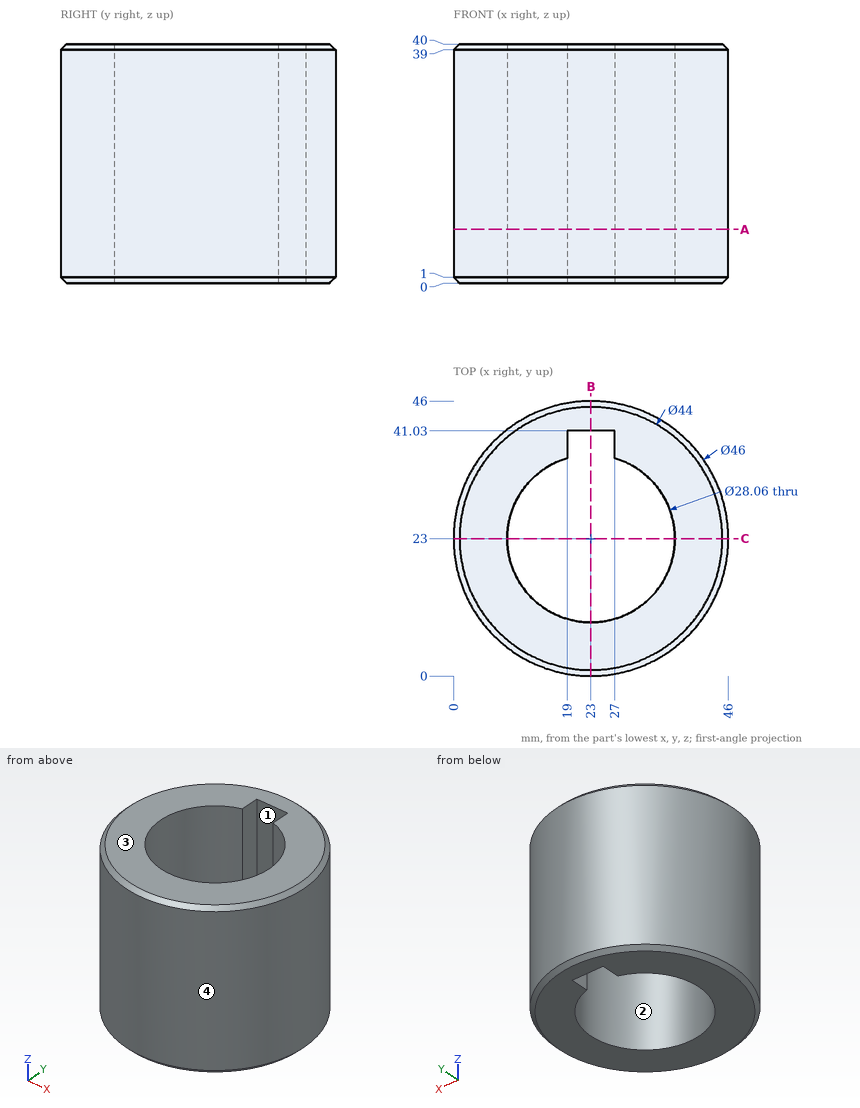
Job drawing, mm, ordinate dimensions from the low corner. One solid piece. Give positions to 0.01 mm unless a question says otherwise; leave off trailing zeros. Loops run counter-clockwise (first coordinate to the right, second up) from the corner with the lowest first, then second, coordinate; pieces in that order, holes last. Notation, with made-up numbers: M 54,64 L 66,64 A12 ccw 66,74 Z; hole C -13.75,24.25 d2. An arc over 180 degrees is marked long. Return JSON: item names as keys, results as strings.
1) Saw through at A-A, the plane z = 9. List the corners of the cut face in (x, y).
Calculated:
{"outline": "C 23,23 d46; hole M 19,36.45 A14.03 ccw long 27,36.45 L 27,41.03 L 19,41.03 Z"}
2) Saw through at C-C, the plane y = 23. List the corners of the cut face in (x, z).
Calculated:
{"outline": "M 0,1 L 1,0 L 8.97,0 L 8.97,40 L 1,40 L 0,39 Z; M 37.03,0 L 45,0 L 46,1 L 46,39 L 45,40 L 37.03,40 Z"}
3) Flat gauge pins, fed straight in: pin 1 Ø2 at (y, z) = (31.5, 12) entering from +X; pin 2 Ø5 at (y, z) = (38, 21.5) entering from +X; pin 3 Ø10 at (y, z) = (16.5, 18.5) entering from -X. Where does each tip first touch, or does it go through?
Calculated:
{"pin 1": "stops at x = 44.74", "pin 2": "stops at x = 42.31", "pin 3": "stops at x = 0.05"}
4) Drill centre lines: line 1 (Y direction, x = 23, z = 31); line 2 (Y direction, x = 29, z = 11.5); line 3 (X direction, y = 22, z = 19.5). Where is each one in solid material? Low to high.
Calculated:
{"line 1": "y = 0 to 8.97, 41.03 to 46", "line 2": "y = 0.8 to 10.32, 35.68 to 45.2", "line 3": "x = 0.02 to 9.01, 36.99 to 45.98"}
5) Pull direction X, two halves, no side cores. Call the marked faces 1, 2, 3 and 4: released by +X, released by -X, zero draft, split by the parting line, or undercut.
Calculated:
{"face 1": "undercut", "face 2": "undercut", "face 3": "zero draft", "face 4": "split by the parting line"}
6) Saw through at B-B, the plane x = 23. List the corners of the cut face in (y, z), then the cut area to 3 significant figures.
Calculated:
{"outline": "M 0,1 L 1,0 L 8.97,0 L 8.97,40 L 1,40 L 0,39 Z; M 41.03,0 L 45,0 L 46,1 L 46,39 L 45,40 L 41.03,40 Z", "area": "556 mm2"}
